```python
from build123d import *

# Parameters (mm, degrees)
ESQUISSE1_R             = 28.4
ESQUISSE1_R_2           = 7
BOSS_EXTRU_1_DEPTH      = 26.4
ESQUISSE2_OUTSIDE_W     = 75.71
ESQUISSE2_OUTSIDE_H     = 75.71
ESQUISSE2_OUTSIDE_R     = 15
ENL_V_MAT_EXTRU_1_DEPTH = 20.4
ESQUISSE3_R             = 2.5
ENL_V_MAT_EXTRU_2_DEPTH = 27.4
ENL_V_MAT_EXTRU_3_REACH = 30.4
ESQUISSE4_R             = 4
ESQUISSE5_W             = 5.1
ESQUISSE5_H             = 9.3
ENL_V_MAT_EXTRU_4_DEPTH = 27.4000001
CHANFREIN1_SIZE         = 0.3


with BuildPart() as part:
    # Esquisse1 → Boss.-Extru.1 (new body)
    with BuildSketch(Plane(origin=(0, 0, 0), x_dir=(1, 0, 0), z_dir=(0, 1, 0))):
        Circle(ESQUISSE1_R)
        Circle(ESQUISSE1_R_2, mode=Mode.SUBTRACT)
    extrude(amount=BOSS_EXTRU_1_DEPTH)

    # Esquisse2 outside → Enlèv. mat.-Extru.1 (cut)
    with BuildSketch(Plane(origin=(0, 26.4, 0), x_dir=(1, 0, 0), z_dir=(0, 1, 0))):
        Rectangle(ESQUISSE2_OUTSIDE_W, ESQUISSE2_OUTSIDE_H)
        Circle(ESQUISSE2_OUTSIDE_R, mode=Mode.SUBTRACT)
    extrude(amount=-ENL_V_MAT_EXTRU_1_DEPTH, mode=Mode.SUBTRACT)

    # Esquisse3 → Enlèv. mat.-Extru.2 (cut, through all)
    with BuildSketch(Plane.XZ):
        with Locations((0.409323167, 23.746472465)):
            Circle(ESQUISSE3_R)
        with Locations((20.769709989, 11.518751972)):
            Circle(ESQUISSE3_R)
        with Locations((20.360386822, -12.227720494)):
            Circle(ESQUISSE3_R)
        with Locations((-0.409323167, -23.746472465)):
            Circle(ESQUISSE3_R)
        with Locations((-20.769709989, -11.518751972)):
            Circle(ESQUISSE3_R)
        with Locations((-20.360386822, 12.227720494)):
            Circle(ESQUISSE3_R)
    extrude(amount=-ENL_V_MAT_EXTRU_2_DEPTH, mode=Mode.SUBTRACT)

    # Esquisse4 → Enlèv. mat.-Extru.3 (cut, up to next)
    with BuildSketch(Plane(origin=(0, 0, 0), x_dir=(0, 0, -1), z_dir=(1, 0, 0)), mode=Mode.PRIVATE) as enl_v_mat_extru_3_sk1:
        with Locations((0, 16.2)):
            Circle(ESQUISSE4_R)
    enl_v_mat_extru_3_tool1 = extrude(enl_v_mat_extru_3_sk1.sketch, amount=-ENL_V_MAT_EXTRU_3_REACH, mode=Mode.PRIVATE) & part.part
    add(enl_v_mat_extru_3_tool1.solids().sort_by_distance((0, 16.2, 0))[0], mode=Mode.SUBTRACT)

    # Esquisse5 → Enlèv. mat.-Extru.4 (cut, through all)
    with BuildSketch(Plane(origin=(0, 26.4, 0), x_dir=(1, 0, 0), z_dir=(0, 1, 0))):
        with Locations((0, 4.65)):
            Rectangle(ESQUISSE5_W, ESQUISSE5_H)
    extrude(amount=-ENL_V_MAT_EXTRU_4_DEPTH, mode=Mode.SUBTRACT)

    # Chanfrein1
    chanfrein1_edges = [part.edges().sort_by_distance(p)[0] for p in [
        (-15, 6, 0),
        (-15, 26.4, 0),
        (-28.4, 6, 0),
        (-28.4, 0, 0),
        (0, 26.4, 7),
        (0, 0, 7),
    ]]
    chamfer(chanfrein1_edges, length=CHANFREIN1_SIZE)


solid = part.part
```
Read the model definition and answer for the solid it produces. Units are mm, in the model's axes. A direction names the side the tool comes from. Coordinates: 2 decimals unless noted, no trailing zeros. Order: outer loops, then holes, each group sorted by start corner. A loop starts at its lowest first (then second) coordinate and runs counter-clockwise, first axis right, second up. Notation, with made-up numbers: (81, 44.25) - (99, 44.25) arc R16 ccw to (99, 72.25) - close; hole circle Ø4 at (45, -27). An arc over 180 degrees is marked (long way). Answer as a JSON object with one key per item and string values. Group by question number.
Item 1: Section C-C (y = 9.25) is taken. Give the vertices of the cut face in (x, z), plus the area to 3 significant figures.
Item 2: Consider probe 1 along X at (y, z) = (10.25, 0); probe 2 along Y at (x, z) = (-4, -20.5); probe 3 along X at (y, z) = (9.5, -3). Determine where each line is inside the solid, lowest interval first. Write a range as from..to.
Item 3: Section A-A (z = 0) is taken. Give the vertices of the cut face in (x, y), plus the area to 3 significant figures.
Item 4: A tool of negligible diameter and unlimited length cuts with its end or side. For faces 4 (the face through (-0.277, 26.219, 7.113)), 5 (the face through (-2.55, 13, -8)), 6 (the face through (-10.311, 17.401, -3.815)), from which of +Z, -Z, +X, -X, +Y, -Y can it reach the whole face along a straight path? Write none if from no direction.
Item 5: Section D-D (y = 4.25) is taken. Give the vertices of the cut face in (x, z), plus the area to 3 significant figures.
Item 6: The mould has two halves that part along Z. Classify faces 1 (the face through (12, 6, 12)), 2 (the face through (13.856, 16.339, 5.745)), 3 (the face through (-22.858, 2.958, 12.338)): +Z half, -Z half, draft (parallel to the pull), parting line (faces both ways), or undercut.
Item 7: Flat-ended cylindrical pins translate along their axes: P1, Ø5, axis at y = 3.5, z = 13, coming from the +X side; P2, Ø8, axis at y = 5.5, z = -18.5, coming from the -X side; P3, Ø8, axis at x = -0.41, z = -23.75, coming from the +Y side. Find the tip coordinate at first contact, or state that the pin passes through.
Item 8: Section B-B (x = 0) is taken. State how many separate pieces and enclosed holes the cut face has, plus the area to 3 significant figures.
Results are:
{
 "1": {"outline": "circle Ø30 at (0, 0); hole (-2.55, -9.3) - (2.55, -9.3) - (2.55, -6.52) arc R7 ccw (long way) to (-2.55, -6.52) - close", "area": "540 mm^2"},
 "2": {"probe 1": "x = -15..-7, 7..15", "probe 2": "y = 0..6", "probe 3": "x = -14.7..-6.32, 6.32..14.7"},
 "3": {"outline": "(-28.4, 0.3) - (-28.1, 0) - (-7.3, 0) - (-7, 0.3) - (-7, 12.2) - (-15, 12.2) - (-15, 6.3) - (-15.3, 6) - (-28.1, 6) - (-28.4, 5.7) - close; (-15, 20.2) - (-7, 20.2) - (-7, 26.1) - (-7.3, 26.4) - (-14.7, 26.4) - (-15, 26.1) - close; (7, 0.3) - (7.3, 0) - (28.1, 0) - (28.4, 0.3) - (28.4, 5.7) - (28.1, 6) - (15.3, 6) - (15, 6.3) - (15, 26.1) - (14.7, 26.4) - (7.3, 26.4) - (7, 26.1) - close", "area": "519 mm^2"},
 "4": {"face 4": "+Y", "face 5": "+Y, -Y", "face 6": "-X"},
 "5": {"outline": "circle Ø56.8 at (0, 0); hole circle Ø5 at (-20.77, -11.52); hole circle Ø5 at (-20.36, 12.23); hole circle Ø5 at (-0.41, -23.75); hole (-2.55, -9.3) - (2.55, -9.3) - (2.55, -6.52) arc R7 ccw (long way) to (-2.55, -6.52) - close; hole circle Ø5 at (0.41, 23.75); hole circle Ø5 at (20.36, -12.23); hole circle Ø5 at (20.77, 11.52)", "area": "2,250 mm^2"},
 "6": {"face 1": "draft", "face 2": "parting line", "face 3": "undercut"},
 "7": {"P1": "stops at x = 26.39", "P2": "stops at x = -24.42", "P3": "stops at y = 6"},
 "8": {"separate pieces": "4", "enclosed holes": "0", "area": "463 mm^2"}
}
